Could you check a few things on this model? Use its own coordinates, in mm. A direction names the side the tool comes from. Coordinates: 2 decimals unless noted, no trailing zeros. Loops run counter-clockwise (first coordinate to the right, second up) from the corner with the lowest first, then second, coordinate; pieces in that order, holes last. Notation, with made-up numbers: (66, 84) -> (116, 84) arc R5 ccw to (116, 88) -> close; hole circle Ø10 at (46.25, -3). An arc over 180 degrees is marked (long way). One line per question, with ' | ' between items.
Autodesk Inventor part; units mm, degrees
ref_plane "YZ Plane" through (0, 0, 0) normal (1, 0, 0) x (0, 1, 0)
ref_plane "XZ Plane" through (0, 0, 0) normal (0, 1, 0) x (-1, 0, 0)
ref_plane "XY Plane" through (0, 0, 0) normal (0, 0, 1) x (1, 0, 0)
sketch "Sketch1" plane through (0, 0, 0) normal (0, 0, 1) x (1, 0, 0)
  circle A0 centre (0, 0) radius 9.5
  circle A1 centre (-11, 0) radius 3.25
  circle A2 centre (11, 0) radius 3.25
  line L0 (-11, 3.25) -> (11, 3.25)
  line L1 (11, 3.25) -> (11, -3.25)
  line L2 (11, -3.25) -> (-11, -3.25)
  line L3 (-11, -3.25) -> (-11, 3.25)
  dimension "d15" = 6.5
  dimension "d17" = 6.5
  dimension "d12" = 19
  dimension "d16" = 11
  dimension "d18" = 11
extrude "Extrusion1" add sketch "Sketch1" along normal blind 6
sketch "草圖4" plane through (0, 0, 6) normal (0, 0, 1) x (1, 0, 0)
  arc A0 (-8.9268, -3.25) -> (8.9268, -3.25) centre (0, 0) ccw
  circle A1 centre (0, 0) radius 6
  line L0 (-6, 0) -> (6, 0)
  line L1 (6, 0) -> (6, -9.5)
  line L2 (6, -9.5) -> (-6, -9.5)
  line L3 (-6, -9.5) -> (-6, 0)
  line L4 (-8, -9.5) -> (8, -9.5)
  line L5 (8, -9.5) -> (8, -6)
  line L6 (8, -6) -> (-8, -6)
  line L7 (-8, -6) -> (-8, -9.5)
  dimension "d19" = 12
  dimension "d23" = 6
  dimension "d24" = 3.5
  dimension "d26" = 16
  dimension "d27" = 8
extrude "擠出2" cut sketch "草圖4" against normal through all
fillet "圓角2" radius 2 4 edges at (8.9268, -3.25, 3) (-8.9268, -3.25, 3) (8.9268, 3.25, 3) (-8.9268, 3.25, 3)
sketch "草圖5" plane through (0, 0, 6) normal (0, 0, 1) x (1, 0, 0)
  arc A0 (14.25, 0) -> (11, 3.25) centre (11, 0) ccw
  arc A1 (-11, 3.25) -> (-11, -3.25) centre (-11, 0) ccw
hole "孔2" at (-11, 0, 6) at (11, 0, 6) direction (0, 0, -1) diameter 3 end through all
properties part number "plastic_part_13"
Q1. Imagine slicing it at C-C on x = 0. Write out the boundary of the cut face in (y, z).
Values follow:
outline: (6, 0) -> (9.5, 0) -> (9.5, 6) -> (6, 6) -> close
Q2. Please list where these lines run through material, in increasing order: L1, parallel to X at y = 0, z = 1.3; L2, parallel to Y at x = 11, z = 2.75; L3, parallel to X at y = 1, z = 5.7. Write a range as [from, to].
Values follow:
L1: x = [-14.25, -12.5], [-9.5, -6], [6, 9.5], [12.5, 14.25] | L2: y = [-3.25, -1.5], [1.5, 3.25] | L3: x = [-14.09, -12.12], [-9.88, -5.92], [5.92, 9.88], [12.12, 14.09]
Q3. For faces 1 (the face through (6, -3, 3)), 2 (the face through (-7, -6, 3)), which set-ups out of +Z, -Z, +X, -X, +Y, -Y let a thin tool reach every point of the face, with its end or its side?
Values follow:
face 1: +Z, -Z, -Y | face 2: +Z, -Z, +X, -X, -Y
Q4. Imagine slicing it at D-D on y = -2. Write out the boundary of the cut face in (x, z).
Values follow:
outline: (-13.56, 0) -> (-6, 0) -> (-6, 6) -> (-13.56, 6) -> close; (6, 0) -> (13.56, 0) -> (13.56, 6) -> (6, 6) -> close
Q5. Imagine slicing it at A-A on z = 2.8. Write out the boundary of the cut face in (x, y), plus the area to 3 significant figures.
Values follow:
outline: (-11, -3.25) -> (-10.23, -3.25) arc R2 cw to (-8.45, -4.34) arc R9.5 ccw to (-7.37, -6) -> (-6, -6) -> (-6, 0) arc R6 cw to (6, 0) -> (6, -6) -> (7.37, -6) arc R9.5 ccw to (8.45, -4.34) arc R2 cw to (10.23, -3.25) -> (11, -3.25) arc R3.25 ccw to (11, 3.25) -> (10.23, 3.25) arc R2 cw to (8.45, 4.34) arc R9.5 ccw to (-8.45, 4.34) arc R2 cw to (-10.23, 3.25) -> (-11, 3.25) arc R3.25 ccw to start; hole circle Ø3 at (-11, 0); hole circle Ø3 at (11, 0) | area: 161 mm2
Q6. Imagine slicing it at B-B on y = -5. Write out the boundary of the cut face in (x, z), plus the area to 3 significant figures.
Values follow:
outline: (-8.08, 0) -> (-6, 0) -> (-6, 6) -> (-8.08, 6) -> close; (6, 0) -> (8.08, 0) -> (8.08, 6) -> (6, 6) -> close | area: 24.9 mm2
Q7. We'd pull the mould along X, two halves only. Please class faces 3 (the face through (-7.945, -5.209, 2.958)), 4 (the face through (7, -6, 3)), 5 (the face through (-9.536, 0.325, 2.958)), 6 (the face through (-0.1, 9.5, 3)): released by +X, released by -X, zero draft, split by the parting line, or undercut.
Values follow:
face 3: released by -X | face 4: zero draft | face 5: undercut | face 6: split by the parting line
Q8. For pin 1 (1.5 mm diameter, centred on x = -6.5, z = 4, fed in from +Y); pin 2 (0.8 mm diameter, centred on x = 10.5, z = 4.5, fed in from -Y); pin 3 (0.6 mm diameter, centred on x = 10.5, z = 2.5, fed in from +Y), each with a flat end and sliding along its axis, tell me the tip position at first contact or that it passes through.
Values follow:
pin 1: stops at y = 7.56 | pin 2: stops at y = -3.25 | pin 3: stops at y = 3.25
